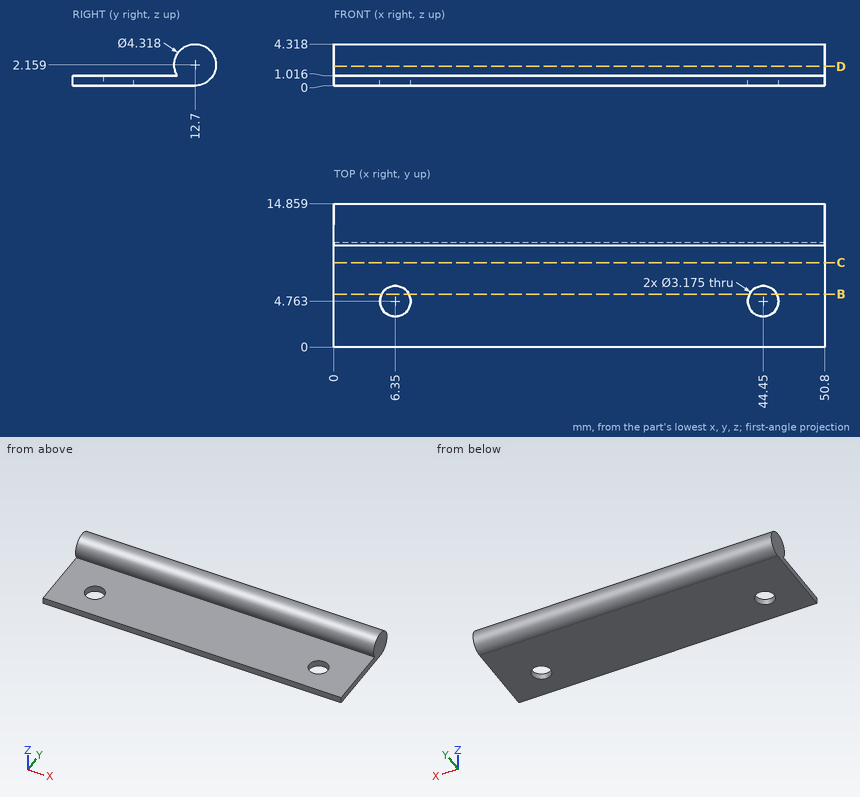
Study the drawing (mm; zero at the part's minimum x, y, z) and answer. Round coordinates to 2 decimals unless told otherwise and drop trailing zeros. Order: outer loops, then holes, each group sorted by start corner. A loop starts at its lowest first (then second) coordinate and runs counter-clockwise, first axis right, second up. Notation, with made-up numbers: (38, 17.25) -> (50, 17.25) arc R12 cw to (50, 34.25) -> close; hole circle Ø10 at (8.5, 68.25). An arc over 180 degrees is marked (long way). Answer as CSV lines item,"result". Start each with the question number.
(1) The part is cut by section B-B (y = 5.5). Determine the outline of the cut face in (x, z) (1 decimal).
(2) Flat-ended cylindrical pins translate along their axes: pin 1 Ø6 at (x, y) = (6.5, 9) entering from +Z; pin 2 Ø5 at (x, y) = (44.45, 4.76) entering from +Z; pin 3 Ø2.5 at (x, y) = (6.35, 4.76) entering from +Z; pin 4 Ø2 at (x, z) = (21, 3.5) entering from +Y. Find the tip coordinate at first contact, or state that the pin passes through.
(3) The part is cut by section C-C (y = 8.75). Determine the outline of the cut face in (x, z) (1 decimal).
(4) The part is cut by section D-D (z = 2). Determine the outline of the cut face in (x, y), then the cut area to 3 significant figures.
(5) Find the intervals of material crossed by probe 1 along X at (y, z) = (4.75, 0.65); probe 2 along Z at (x, y) = (41.5, 2) (1 decimal); probe 3 along Z at (x, y) = (9.5, 12.5), in increasing order. Write a range as from..to.
Evaluation:
1,outline,"(0, 0) -> (4.9, 0) -> (4.9, 1) -> (0, 1) -> close; (7.8, 0) -> (43, 0) -> (43, 1) -> (7.8, 1) -> close; (45.9, 0) -> (50.8, 0) -> (50.8, 1) -> (45.9, 1) -> close"
2,pin 1,"z = 4.2"
2,pin 2,"z = 1.02"
2,pin 3,"through"
2,pin 4,"y = 14.83"
3,outline,"(0, 0) -> (50.8, 0) -> (50.8, 1) -> (0, 1) -> close"
4,outline,"(0, 10.55) -> (50.8, 10.55) -> (50.8, 14.85) -> (0, 14.85) -> close"
4,area,"219 mm²"
5,probe 1,"0..4.76, 7.94..42.86, 46.04..50.8"
5,probe 2,"0..1"
5,probe 3,"0..4.31"
